Verification items for the finished model (mm, model axes). Round coordinates to 2 decimals unless told otherwise and drop trailing zeros. Write each loop counter-clockwise with the first axis right and the second up, starting at its lowest first coordinate (ties: lowest second). Pieces come first, ordered by that corner, then holes. Notation, with made-up numbers: (5.25, -34) - (38.25, -34) arc R12 cw to (38.25, -16) - close; hole circle Ø7 at (34.25, 65). An arc over 180 degrees is marked (long way). Answer as a JSON object with one key per item and string values. Group by question number.
1) Section check B-B (z = -3). Enter the section's corners in (x, y).
2) Mould release check, pull along X, two halves, no side actions. Record for faces 1 (the cylindrical face through (-4, -27.6, 1.7)), 2 (the flat face through (4, -27, 0)), 3 (the cylindrical face through (-0.208, -25.914, -1.972)), 4 (the cylindrical face through (7.774, -24.92, 0.493)): +X half, -X half, draft (parallel to the pull), parting line (faces both ways), or undercut.
3) Section check A-A (z = 1.25). Enter the section's corners in (x, y), then the cut area to 3 significant figures.
4) Go/stop test with flat-tipped pins: pin 1 Ø1 at (x, y) = (3.5, -30.5) entering from -Z; pin 2 Ø5 at (x, y) = (8.95, -26) entering from +Z; pin 3 Ø4 at (y, z) = (-29.5, -3) entering from +X. Record where each tip stops, or that it passes through.
5) Thickness scan on line 1 (Z direction, x = -2, y = -29.25); line 2 (Y direction, x = 9, z = 0.5); line 3 (X direction, y = -25.75, z = 1.5). Record the ranges inside material, lowest first.
6) Section check D-D (z = 2.75). Enter the section's corners in (x, y), then the cut area to 3 significant figures.
7) Section check C-C (y = -30.5). Enter the section's corners in (x, z).
```python
from build123d import *

# Parameters (mm, degrees)
SKETCH_1_R          = 1.6
EXTRUDE_1_DEPTH     = 4
SKETCH_2_R          = 1.6
EXTRUDE_2_DEPTH     = 4
CUT_EXTRUDE_START   = -0.5
CUT_EXTRUDE_1_DEPTH = 0.5


with BuildPart() as part:
    # 草图1 → 凸台-拉伸1 (new body)
    with BuildSketch(Plane.XY):
        with BuildLine():
            ThreePointArc((-0.416971099, -23.521792476), (-3.994548166, -27.708770095), (0, -31.5))
            ThreePointArc((0, -31.5), (5.198999585, -31.067996448), (10.255396865, -29.783835131))
            ThreePointArc((10.255396865, -29.783835131), (12.798012634, -24.898659157), (8.052200486, -22.104539206))
            ThreePointArc((8.052200486, -22.104539206), (3.83936707, -22.943152918), (-0.416971099, -23.521792476))
        make_face()
        with Locations((8.953124248, -26.001760829)):
            Circle(SKETCH_1_R, mode=Mode.SUBTRACT)
    extrude(amount=EXTRUDE_1_DEPTH)

    # 草图2 → 凸台-拉伸2 (add)
    with BuildSketch(Plane.XY):
        with Locations((0, -27.5)):
            Circle(SKETCH_2_R)
    extrude(amount=-EXTRUDE_2_DEPTH)

    # 草图3 → 切除-旋转1 (revolve, cut)
    with BuildSketch(Plane(origin=(0, -26.001760829, 0), x_dir=(1, 0, 0), z_dir=(0, 1, 0))):
        Polygon((8.953124248, -3.5), (5.853124248, -3.5), (7.353124248, -1), (8.953124248, -1), align=None)
    revolve(axis=Axis((8.953124248, -26.001760829, 1), (0, 0, 1)), mode=Mode.SUBTRACT)

    # 草图5 → 切除-拉伸1 (cut)
    with BuildSketch(Plane.XY.offset(4).offset(CUT_EXTRUDE_START)):
        with BuildLine():
            ThreePointArc((-0.416971099, -23.521792476), (-3.994548166, -27.708770095), (0, -31.5))
            ThreePointArc((0, -31.5), (5.198999585, -31.067996448), (10.255396865, -29.783835131))
            ThreePointArc((10.255396865, -29.783835131), (12.798012634, -24.898659157), (8.052200486, -22.104539206))
            ThreePointArc((8.052200486, -22.104539206), (3.83936707, -22.943152918), (-0.416971099, -23.521792476))
        make_face()
    extrude(amount=CUT_EXTRUDE_1_DEPTH, mode=Mode.SUBTRACT)


solid = part.part
```
Returned:
{
 "1": {"outline": "circle Ø3.2 at (0, -27.5)"},
 "2": {"face 1": "-X half", "face 2": "draft", "face 3": "parting line", "face 4": "undercut"},
 "3": {"outline": "(-0.42, -23.52) arc R4 ccw to (0, -31.5) arc R31.5 ccw to (10.26, -29.78) arc R4 ccw to (8.05, -22.1) arc R70 cw to start; hole circle Ø3.5 at (8.95, -26)", "area": "115 mm2"},
 "4": {"pin 1": "z = 0", "pin 2": "z = 2.51", "pin 3": "x = 1.6"},
 "5": {"line 1": "0 to 3.5", "line 2": "-30.19 to -27.6, -24.4 to -22", "line 3": "-3.6 to 7.07, 10.84 to 12.95"},
 "6": {"outline": "(-0.42, -23.52) arc R4 ccw to (0, -31.5) arc R31.5 ccw to (10.26, -29.78) arc R4 ccw to (8.05, -22.1) arc R70 cw to start; hole circle Ø5.3 at (8.95, -26)", "area": "102 mm2"},
 "7": {"outline": "(-2.65, 0) - (7.87, 0) - (7.87, 3.5) - (-2.65, 3.5) - close"}
}
